The model under review builds one solid part; all positions refer to its coordinate system, in mm. Round coordinates to 2 decimals unless told otherwise and drop trailing zeros. Order: outer loops, then holes, each group sorted by start corner. A loop starts at its lowest first (then second) coordinate and runs counter-clockwise, first axis right, second up.
1) To check wall thickness, follow L1, parallel to X at y = 0.75, z = 0; L2, parallel to X at y = 0.5, z = -35; L3, parallel to X at y = 0.4, z = 33. State the ranges of each line that lie inside material, in increasing order.
2) Consider section D-D (z = 24.5). Give the boundary of the cut face in (x, y), then the cut area to 3 significant figures.
3) Clearance check with flat-ended pins moving along their axes: P1, Ø0.5, axis at x = 32.5, y = 0.5, coming from the +Z side; P2, Ø0.5, axis at x = -32.5, y = 0.5, coming from the -Z side. State where each tip first meets the part, or that it passes through.
4) Consider section C-C (y = 0.85). Give the boundary of the cut face in (x, z).
5) Consider section B-B (z = -35). Give the boundary of the cut face in (x, y), then the cut area to 3 significant figures.
6) Consider section A-A (z = 0). Give the boundary of the cut face in (x, y).
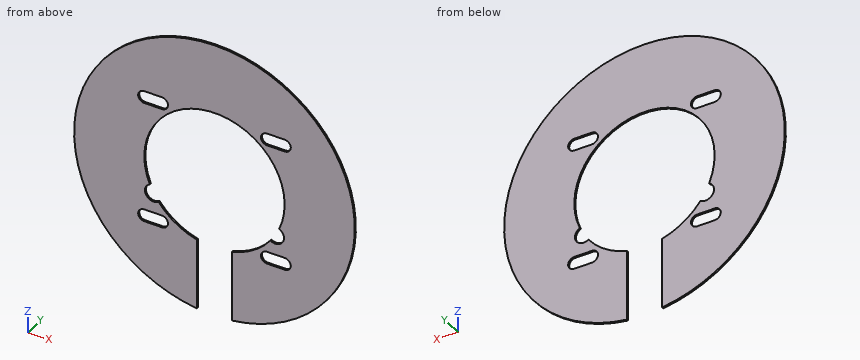
from build123d import *

# Parameters (mm, degrees)
EXTRUDE_1_DEPTH     = 1
CUT_EXTRUDE_1_DEPTH = 1
SKETCH_4_R          = 5
CUT_EXTRUDE_2_DEPTH = 1


with BuildPart() as part:
    # 草图1 → 凸台-拉伸1 (new body)
    with BuildSketch(Plane(origin=(0, 0, 0), x_dir=(1, 0, 0), z_dir=(0, 1, 0))):
        with BuildLine():
            Line((-10, 79.372539332), (-10, 38.729833462))
            ThreePointArc((-10, 38.729833462), (0, -40), (10, 38.729833462))
            Line((10, 38.729833462), (10, 79.372539332))
            ThreePointArc((10, 79.372539332), (0, -80), (-10, 79.372539332))
        make_face()
    extrude(amount=EXTRUDE_1_DEPTH)

    # 草图2 → 切除-拉伸1 (cut)
    with BuildSketch(Plane(origin=(0, 1, 0), x_dir=(1, 0, 0), z_dir=(0, 1, 0))):
        with BuildLine():
            Line((-40, 38.5), (-30, 38.5))
            ThreePointArc((-30, 38.5), (-26.5, 35), (-30, 31.5))
            Line((-30, 31.5), (-40, 31.5))
            ThreePointArc((-40, 31.5), (-43.5, 35), (-40, 38.5))
        make_face()
        with BuildLine():
            Line((30, 38.5), (40, 38.5))
            ThreePointArc((40, 38.5), (43.5, 35), (40, 31.5))
            Line((40, 31.5), (30, 31.5))
            ThreePointArc((30, 31.5), (26.5, 35), (30, 38.5))
        make_face()
        with BuildLine():
            Line((30, -31.5), (40, -31.5))
            ThreePointArc((40, -31.5), (43.5, -35), (40, -38.5))
            Line((40, -38.5), (30, -38.5))
            ThreePointArc((30, -38.5), (26.5, -35), (30, -31.5))
        make_face()
        with BuildLine():
            Line((-40, -31.5), (-30, -31.5))
            ThreePointArc((-30, -31.5), (-26.5, -35), (-30, -38.5))
            Line((-30, -38.5), (-40, -38.5))
            ThreePointArc((-40, -38.5), (-43.5, -35), (-40, -31.5))
        make_face()
    extrude(amount=-CUT_EXTRUDE_1_DEPTH, mode=Mode.SUBTRACT)

    # 草图4 → 切除-拉伸2 (cut)
    with BuildSketch(Plane(origin=(0, 1, 0), x_dir=(1, 0, 0), z_dir=(0, 1, 0))):
        with Locations((34.641016151, 20)):
            Circle(SKETCH_4_R)
        with Locations((-34.641016151, 20)):
            Circle(SKETCH_4_R)
    extrude(amount=-CUT_EXTRUDE_2_DEPTH, mode=Mode.SUBTRACT)


solid = part.part
Answer below:
1. L1: x = -80 to -40, 40 to 80
1. L2: x = -71.94 to -43.5, -26.5 to -19.36, 19.36 to 26.5, 43.5 to 71.94
1. L3: x = -72.88 to -42.87, -27.13 to -22.61, 22.61 to 27.13, 42.87 to 72.88
2. outline: (-76.16, 0) - (-31.62, 0) - (-31.62, 1) - (-76.16, 1) - close; (31.62, 0) - (76.16, 0) - (76.16, 1) - (31.62, 1) - close
2. area: 89.1 mm2
3. P1: stops at z = 73.21
3. P2: stops at z = -73.21
4. outline: (-36.87, -15.52) arc R40 cw (long way) to (36.87, -15.52) arc R5 cw (long way) to (31.88, -24.17) arc R40 cw to (10, -38.73) - (10, -79.37) arc R80 ccw (long way) to (-10, -79.37) - (-10, -38.73) arc R40 cw to (-31.88, -24.17) arc R5 cw (long way) to start; hole (-40, -38.5) - (-30, -38.5) arc R3.5 ccw to (-30, -31.5) - (-40, -31.5) arc R3.5 ccw to start; hole (-40, 31.5) - (-30, 31.5) arc R3.5 ccw to (-30, 38.5) - (-40, 38.5) arc R3.5 ccw to start; hole (30, -38.5) - (40, -38.5) arc R3.5 ccw to (40, -31.5) - (30, -31.5) arc R3.5 ccw to start; hole (30, 31.5) - (40, 31.5) arc R3.5 ccw to (40, 38.5) - (30, 38.5) arc R3.5 ccw to start
5. outline: (-71.94, 0) - (-43.5, 0) - (-43.5, 1) - (-71.94, 1) - close; (-26.5, 0) - (-19.36, 0) - (-19.36, 1) - (-26.5, 1) - close; (19.36, 0) - (26.5, 0) - (26.5, 1) - (19.36, 1) - close; (43.5, 0) - (71.94, 0) - (71.94, 1) - (43.5, 1) - close
5. area: 71.1 mm2
6. outline: (-80, 0) - (-40, 0) - (-40, 1) - (-80, 1) - close; (40, 0) - (80, 0) - (80, 1) - (40, 1) - close
